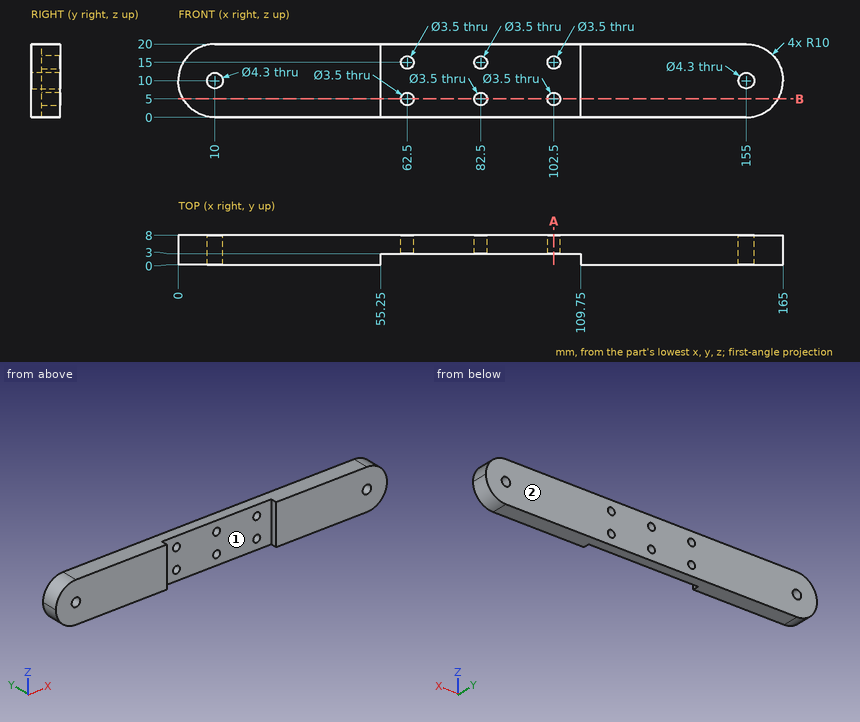
Could you check a few things on this drawing? It's one solid part, dimensions in mm from its lowest x, y, z. A direction names the side the tool comes from. Coordinates: 2 decimals unless noted, no trailing zeros. Write each loop counter-clockwise with the first axis right and the second up, starting at its lowest first coordinate (ties: lowest second). Pieces come first, ordered by that corner, then holes. Notation, with made-up numbers: M -39.75,86 L 6.25,86 A28 ccw 6.25,124 Z; hole C 72,19.25 d4. An arc over 180 degrees is marked long. Answer as CSV lines item,"result". Start each with the question number.
Q1. For the marked faces 1 and 2, which set-ups out of +Z, -Z, +X, -X, +Y, -Y let a thin tool reach every point of the face, with its end or its side?
Q2. I need wall thicknesses on probe 1 along X at (y, z) = (3.5, 10); probe 2 along X at (y, z) = (2.25, 10); probe 3 along Z at (x, y) = (102.5, 5.7). Which ranges of each line are inside material? Lowest first, please. Write a range as [from, to].
Q3. Will these pins go through, and if not, where does the flat tip stop? pin 1 Ø3.5 at (y, z) = (1, 9) entering from +X; pin 2 Ø3 at (x, z) = (82.5, 15) entering from +Y; pin 3 Ø0.9 at (y, z) = (1, 7) entering from -X; pin 4 Ø6 at (x, z) = (87, 9) entering from -Y.
Q4. Suppose I cut it at A-A, the plane x = 102.5. List the corners of the cut face in (y, z) for me, then the cut area to 3 significant figures.
Q5. Suppose I cut it at B-B, the plane z = 5. List the corners of the cut face in (x, y) for me.
Entries:
1,face 1,"+Z, -Z, -Y"
1,face 2,"+Z, -Z, +X, -X, +Y"
2,probe 1,"x = [0, 7.85], [12.15, 152.85], [157.15, 165]"
2,probe 2,"x = [0, 7.85], [12.15, 55.25], [109.75, 152.85], [157.15, 165]"
2,probe 3,"z = [0, 3.25], [6.75, 13.25], [16.75, 20]"
3,pin 1,"stops at x = 165"
3,pin 2,"passes through"
3,pin 3,"stops at x = 0.33"
3,pin 4,"stops at y = 3"
4,outline,"M 3,0 L 8,0 L 8,3.25 L 3,3.25 Z; M 3,6.75 L 8,6.75 L 8,13.25 L 3,13.25 Z; M 3,16.75 L 8,16.75 L 8,20 L 3,20 Z"
4,area,"65.0 mm²"
5,outline,"M 1.34,0 L 55.25,0 L 55.25,3 L 60.75,3 L 60.75,8 L 1.34,8 Z; M 64.25,3 L 80.75,3 L 80.75,8 L 64.25,8 Z; M 84.25,3 L 100.75,3 L 100.75,8 L 84.25,8 Z; M 104.25,3 L 109.75,3 L 109.75,0 L 163.66,0 L 163.66,8 L 104.25,8 Z"
